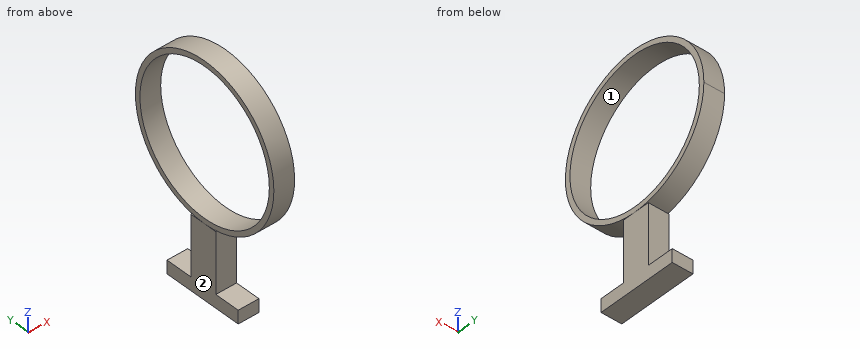
from build123d import *

# Parameters (mm, degrees)
F0_W          = 0.7400371833
F0_H          = 2.6144962758
F1_DEPTH      = 1
F3_W          = 0.7400371833
F3_H          = 0.471592648
F4_DEPTH      = 0.96
F4_DEPTH_BACK = 1.9
F5_R          = 2.5243511124
F6_DEPTH      = 0.37
F6_DEPTH_BACK = 0.37
F7_R          = 2.7819768233
F8_DEPTH      = 0.37
F9_R          = 2.6
F10_DEPTH     = 2.5


with BuildPart() as f1:
    # F0 (on Front) → F1 (new body)
    with BuildSketch(Plane.XZ):
        Rectangle(F0_W, F0_H)
    extrude(amount=F1_DEPTH)

    # F3 (on face) → F4 (join, two sides)
    with BuildSketch(Plane(origin=(0, 0, 0), x_dir=(-1, 0, 0), z_dir=(0, 1, 0))) as f4_sk:
        with Locations((0, -1.0714518139)):
            Rectangle(F3_W, F3_H)
    extrude(amount=F4_DEPTH)
    extrude(f4_sk.sketch, amount=-F4_DEPTH_BACK)

    # F5 (on Right) → F6 (cut, two sides)
    with BuildSketch(Plane.YZ) as f6_sk:
        with Locations((-0.5211759007, 3.8327652696)):
            Circle(F5_R)
    extrude(amount=-F6_DEPTH, mode=Mode.SUBTRACT)
    extrude(f6_sk.sketch, amount=F6_DEPTH_BACK, mode=Mode.SUBTRACT)

    # F7 (on Right) → F8 (join, symmetric)
    with BuildSketch(Plane.YZ):
        with Locations((-0.550427369, 4.088926369)):
            Circle(F7_R)
    extrude(amount=F8_DEPTH, both=True)

    # F9 (on face) → F10 (cut)
    with BuildSketch(Plane.YZ.offset(0.37)):
        with Locations((-0.550427369, 4.088926369)):
            Circle(F9_R)
    extrude(amount=-F10_DEPTH, mode=Mode.SUBTRACT)


solid = f1.part
Source: CAD feature listing. Evaluate the final solid. Frame: model axes, mm. Face numbers are marked on the shaded views. Round coordinates to 2 decimals unless told otherwise and drop trailing zeros. Loops run counter-clockwise (first coordinate to the right, second up) from the corner with the lowest first, then second, coordinate; pieces in that order, holes last. Notation, with made-up numbers: (24.5, 16) - (82.5, 16) arc R7 ccw to (82.5, 22) - close; hole circle Ø4 at (40, -23). An arc over 180 degrees is marked (long way). Write item = value, one per line. Start each with the question number.
(1) Section query C-C, the plane x = 0.1. Output: boundary loops of the cut face in (y, z).
(2) Section query B-B, the plane z = 2.25. Output: boundary loops of the cut face in (x, y).
(3) Ray query, line 1 along Y through (x, z) = (-0.05, -1); line 2 along Z through (x, y) = (0.1, 0.65); line 3 along Y through (x, z) = (-0.2, 4.75). Return the intervals inside material, ascending. Write a range as from..to.
(4) Section query A-A, the plane y = -0.3. Output: boundary loops of the cut face in (x, z).
(5) Section query D-D, the plane y = 1.15. Output: boundary loops of the cut face in (x, z), plus the area to 3 significant figures.
(6) Pin query (flat end, axial travel): pin 1 (3 mm diameter, centred on y = -0.55, z = 4.09, fed in from +X). Return the tip coordinate at first contact, or that it passes through.
(7) Pull-direction query (Z, two-part tool) for the marked faces 1 and 2; classes: +Z half, -Z half, draft (parallel to the pull), parting line (faces both ways), or undercut.
Conclusion:
q1.outline = (-1.9, -1.31) - (0.96, -1.31) - (0.96, -0.84) - (0, -0.84) - (0, 1.31) - (-0.51, 1.31) arc R2.78 ccw (long way) to (-0.59, 1.31) - (-1, 1.31) - (-1, -0.84) - (-1.9, -0.84) - close; hole circle Ø5.2 at (-0.55, 4.09)
q2.outline = (-0.37, -2.64) - (0.37, -2.64) - (0.37, -2.39) - (-0.37, -2.39) - close; (-0.37, 1.29) - (0.37, 1.29) - (0.37, 1.54) - (-0.37, 1.54) - close
q3.line_1 = -1.9..0.96
q3.line_2 = -1.31..-0.84, 1.58..1.78, 6.4..6.6
q3.line_3 = -3.25..-3.06, 1.96..2.15
q4.outline = (-0.37, -1.31) - (0.37, -1.31) - (0.37, 1.31) - (-0.37, 1.31) - close; (-0.37, 1.32) - (0.37, 1.32) - (0.37, 1.5) - (-0.37, 1.5) - close; (-0.37, 6.68) - (0.37, 6.68) - (0.37, 6.86) - (-0.37, 6.86) - close
q5.outline = (-0.37, 1.89) - (0.37, 1.89) - (0.37, 2.12) - (-0.37, 2.12) - close; (-0.37, 6.06) - (0.37, 6.06) - (0.37, 6.29) - (-0.37, 6.29) - close
q5.area = 0.348 mm2
q6.pin_1 = through
q7.face_1 = undercut
q7.face_2 = draft
